Study the drawing (mm; zero at the part's minimum x, y, z) and answer. A direction names the side the tool comes from. Give positions to 0.01 mm unless a question says otherwise; leave off trailing zeros. Order: outer loops, then holes, each group sorted by start corner. A loop starts at its lowest first (then second) coordinate and runs counter-clockwise, first axis right, second up. Notation, with made-up numbers: (76.25, 65) - (118.25, 65) arc R11 ccw to (118.25, 81) - close; hole circle Ø10 at (65, 46.25). An arc over 180 degrees is marked (long way). Write each question's results on one line, items separated by ' | '. Start each with the question number.
1. Section D-D (x = 2.5) is taken. Give the vertices of the cut face in (y, z).
2. A flat-ended cylindrical pin translates along its axis: pin 1 (3.5 mm diameter, centred on x = 14, y = 5, fed in from +Z). Find the tip coordinate at first contact, or state that the pin passes through.
3. Which of the six approach directions +Z, -Z, +X, -X, +Y, -Y give full straight-line access (tool end or side, diameter ignored) to the marked faces 5 and 6?
4. Find the intervals of material crossed by L1, parallel to Y at x = 9, z = 7.6; L2, parallel to X at y = 10, z = 8.9; L3, parallel to Y at x = 8.5, z = 7.5, in increasing order.
5. Section C-C (y = 8.5) is taken. Give the vertices of the cut face in (x, z), and give its area (3 significant figures).
6. Section B-B (x = 14) is taken. Give the vertices of the cut face in (y, z), and give its area (3 significant figures).
7. Section A-A (y = 5) is taken. Give the vertices of the cut face in (x, z), and give its area (3 significant figures).
8. Determine the mould class of the marked faces 1, 2, 3 and 4 for opening direction X: released by +X, released by -X, zero draft, split by the parting line, or undercut.
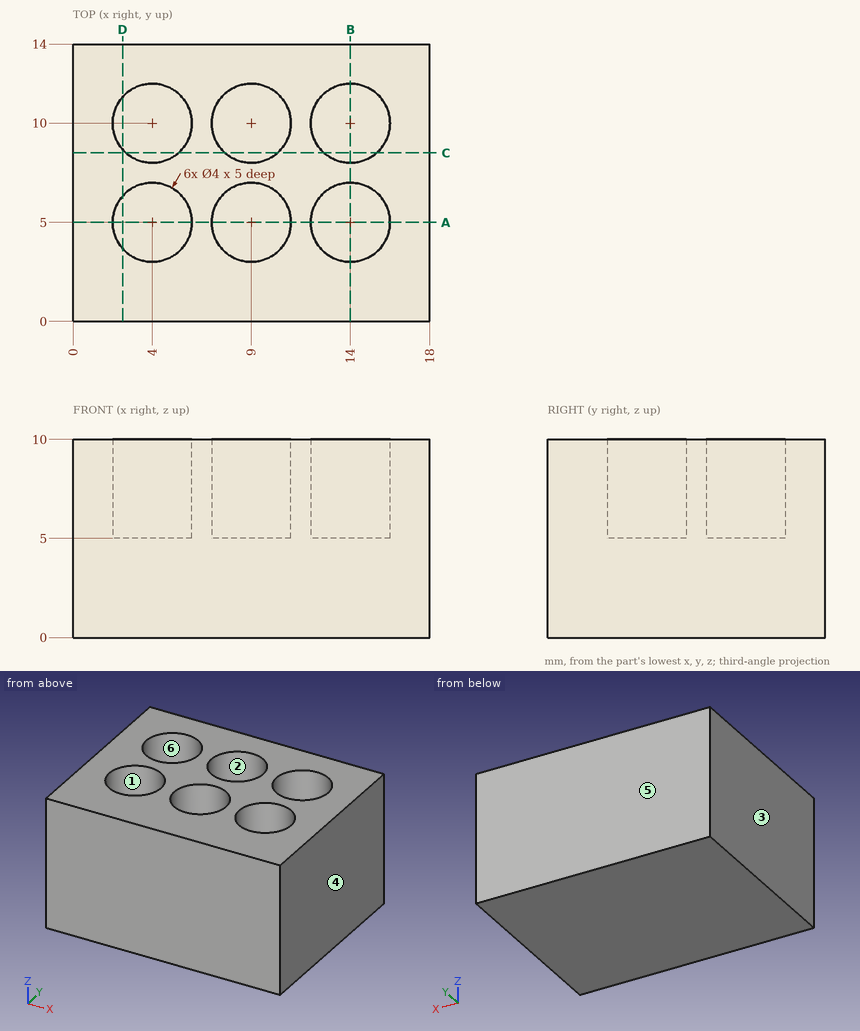
Reported:
1) outline: (0, 0) - (14, 0) - (14, 10) - (11.32, 10) - (11.32, 5) - (8.68, 5) - (8.68, 10) - (6.32, 10) - (6.32, 5) - (3.68, 5) - (3.68, 10) - (0, 10) - close
2) pin 1: z = 5
3) face 5: +Z, -Z, +X, -X, +Y | face 6: +Z
4) L1: 0 to 3, 7 to 8, 12 to 14 | L2: 0 to 2, 6 to 7, 11 to 12, 16 to 18 | L3: 0 to 3.06, 6.94 to 8.06, 11.94 to 14
5) outline: (0, 0) - (18, 0) - (18, 10) - (15.32, 10) - (15.32, 5) - (12.68, 5) - (12.68, 10) - (10.32, 10) - (10.32, 5) - (7.68, 5) - (7.68, 10) - (5.32, 10) - (5.32, 5) - (2.68, 5) - (2.68, 10) - (0, 10) - close | area: 140 mm²
6) outline: (0, 0) - (14, 0) - (14, 10) - (12, 10) - (12, 5) - (8, 5) - (8, 10) - (7, 10) - (7, 5) - (3, 5) - (3, 10) - (0, 10) - close | area: 100 mm²
7) outline: (0, 0) - (18, 0) - (18, 10) - (16, 10) - (16, 5) - (12, 5) - (12, 10) - (11, 10) - (11, 5) - (7, 5) - (7, 10) - (6, 10) - (6, 5) - (2, 5) - (2, 10) - (0, 10) - close | area: 120 mm²
8) face 1: undercut | face 2: undercut | face 3: released by -X | face 4: released by +X
